Geometry: final body of the model. Coordinates: model frame, mm. A direction names the side the tool comes from. Coordinates: 2 decimals unless noted, no trailing zeros. Write each loop counter-clockwise with the first axis right and the second up, starting at its lowest first coordinate (ties: lowest second). Pieces come first, ordered by that corner, then holes.
from build123d import *

# Parameters (mm, degrees)
SKETCH2_R           = 50
BOSS_EXTRUDE1_DEPTH = 5
SKETCH3_R           = 2.5
BOSS_EXTRUDE2_DEPTH = 7
SKETCH4_R           = 50
BOSS_EXTRUDE3_DEPTH = 7


with BuildPart() as part:
    # Sketch2 → Boss-Extrude1 (new body)
    with BuildSketch(Plane(origin=(0, 0, 0), x_dir=(1, 0, 0), z_dir=(0, 1, 0))):
        Circle(SKETCH2_R)
    extrude(amount=BOSS_EXTRUDE1_DEPTH)

    # Sketch3 → Boss-Extrude2 (add)
    with BuildSketch(Plane(origin=(0, 5, 0), x_dir=(1, 0, 0), z_dir=(0, 1, 0))):
        with Locations((40, 0)):
            Circle(SKETCH3_R)
        with Locations((33.650141313, -21.625632698)):
            Circle(SKETCH3_R)
        with Locations((16.61660052, -36.385279814)):
            Circle(SKETCH3_R)
        with Locations((-5.692593531, -39.592857675)):
            Circle(SKETCH3_R)
        with Locations((-26.194429358, -30.229982974)):
            Circle(SKETCH3_R)
        with Locations((-38.379718945, -11.269302274)):
            Circle(SKETCH3_R)
        with Locations((-38.379718945, 11.269302274)):
            Circle(SKETCH3_R)
        with Locations((-26.194429358, 30.229982974)):
            Circle(SKETCH3_R)
        with Locations((-5.692593531, 39.592857675)):
            Circle(SKETCH3_R)
        with Locations((16.61660052, 36.385279814)):
            Circle(SKETCH3_R)
        with Locations((33.650141313, 21.625632698)):
            Circle(SKETCH3_R)
    extrude(amount=BOSS_EXTRUDE2_DEPTH)

    # Sketch4 → Boss-Extrude3 (add)
    with BuildSketch(Plane(origin=(0, 5, 0), x_dir=(1, 0, 0), z_dir=(0, 1, 0))):
        Circle(SKETCH4_R)
        with BuildLine():
            ThreePointArc((44.8625, -3.515123575), (46, 0), (44.8625, 3.515123575))
            ThreePointArc((44.8625, 3.515123575), (43.177183813, 12.677965058), (39.6411559, 21.297388547))
            ThreePointArc((39.6411559, 21.297388547), (38.69766251, 24.869477603), (35.840317333, 27.211608799))
            ThreePointArc((35.840317333, 27.211608799), (29.468733028, 34.008730846), (21.834024893, 39.348130286))
            ThreePointArc((21.834024893, 39.348130286), (19.109090598, 41.843071786), (15.439087149, 42.268600497))
            ThreePointArc((15.439087149, 42.268600497), (6.404167722, 44.541964885), (-2.905254746, 44.90611868))
            ThreePointArc((-2.905254746, 44.90611868), (-6.546482561, 45.531786327), (-9.863944118, 43.905610193))
            ThreePointArc((-9.863944118, 43.905610193), (-18.693675585, 40.933439791), (-26.722136531, 36.206731684))
            ThreePointArc((-26.722136531, 36.206731684), (-30.123593761, 34.76448042), (-32.035242822, 31.602898875))
            ThreePointArc((-32.035242822, 31.602898875), (-37.856408977, 24.328836786), (-42.054928776, 16.011963203))
            ThreePointArc((-42.054928776, 16.011963203), (-44.136676786, 12.959697615), (-44.035578281, 9.266490459))
            ThreePointArc((-44.035578281, 9.266490459), (-45, 0), (-44.035578281, -9.266490459))
            ThreePointArc((-44.035578281, -9.266490459), (-44.136676786, -12.959697615), (-42.054928776, -16.011963203))
            ThreePointArc((-42.054928776, -16.011963203), (-37.856408977, -24.328836786), (-32.035242822, -31.602898875))
            ThreePointArc((-32.035242822, -31.602898875), (-30.123593761, -34.76448042), (-26.722136531, -36.206731684))
            ThreePointArc((-26.722136531, -36.206731684), (-18.693675585, -40.933439791), (-9.863944118, -43.905610193))
            ThreePointArc((-9.863944118, -43.905610193), (-6.546482561, -45.531786327), (-2.905254746, -44.90611868))
            ThreePointArc((-2.905254746, -44.90611868), (6.404167722, -44.541964885), (15.439087149, -42.268600497))
            ThreePointArc((15.439087149, -42.268600497), (19.109090598, -41.843071786), (21.834024893, -39.348130286))
            ThreePointArc((21.834024893, -39.348130286), (29.468733028, -34.008730846), (35.840317333, -27.211608799))
            ThreePointArc((35.840317333, -27.211608799), (38.69766251, -24.869477603), (39.6411559, -21.297388547))
            ThreePointArc((39.6411559, -21.297388547), (43.177183813, -12.677965058), (44.8625, -3.515123575))
        make_face(mode=Mode.SUBTRACT)
    extrude(amount=BOSS_EXTRUDE3_DEPTH)


solid = part.part
Item 1: Section D-D, the plane z = 26. Output: boundary loops of the cut face in (x, y), plus the area to 3 significant figures.
Derived:
outline: (-42.71, 0) - (42.71, 0) - (42.71, 12) - (37.76, 12) - (37.76, 5) - (-36.73, 5) - (-36.73, 12) - (-42.71, 12) - close
area: 504 mm2
Item 2: Section A-A, the plane y = 8.75. State how many separate pieces and enclosed holes the cut face has, plus the area to 3 significant figures.
Derived:
separate pieces: 12
enclosed holes: 1
area: 1,660 mm2
Item 3: Pin query (flat end, axial travel): pin 1 (6 mm diameter, centred on x = -32.5, z = -25.5, fed in from +Y); pin 2 (1.5 mm diameter, centred on y = 4, z = 20, fed in from -X); pin 3 (1.5 mm diameter, centred on x = 18, y = 3, fed in from -Z). Return the tip coordinate at first contact, or that it passes through.
Derived:
pin 1: stops at y = 5
pin 2: stops at x = -46.15
pin 3: stops at z = -46.93
Item 4: Material intervals for probe 1 along X at (y, z) = (8.75, 11) (3 decimals); probe 2 along X at (y, z) = (9.5, -39.5); probe 3 along Z at (x, y) = (-39, 7.75), sorted ascending.
Derived:
probe 1: x = -48.775 to -44.374, -40.865 to -35.894, 43.635 to 48.775
probe 2: x = -30.66 to -21.56, -8.19 to -3.19, 21.74 to 30.66
probe 3: z = -31.29 to -22.45, -13.69 to -8.85, 8.85 to 13.69, 22.45 to 31.29
Item 5: Set-up query: faces 1 (the flat face through (40, 12, 0)), 2 (the cylindrical face through (-40.877, 8.451, 11.159)). Return all of +Z, -Z, +X, -X, +Y, -Y with unobstructed straight access to the full face (end or side cutting, diameter ignored); none if empty.
Derived:
face 1: +Z, -Z, +X, -X, +Y
face 2: +Y
Item 6: Section C-C, the plane x = 0. Output: boundary loops of the cut face in (y, z).
Derived:
outline: (0, -50) - (12, -50) - (12, -45) - (5, -45) - (5, 45) - (12, 45) - (12, 50) - (0, 50) - close
Item 7: Section B-B, the plane z = 0. Output: boundary loops of the cut face in (x, y).
Derived:
outline: (-50, 0) - (50, 0) - (50, 12) - (46, 12) - (46, 5) - (42.5, 5) - (42.5, 12) - (37.5, 12) - (37.5, 5) - (-45, 5) - (-45, 12) - (-50, 12) - close
Item 8: Pull-direction query (Z, two-part tool) for faces 3 (the cylindrical face through (-6.598, 8.451, 45.524)), 4 (the flat face through (17, 12, 36)), 5 (the cylindrical face through (-26.52, 8.45, 27.75)); classes: released by +Z, released by -Z, zero draft, split by the parting line, or undercut.
Derived:
face 3: undercut
face 4: zero draft
face 5: undercut
